from build123d import *

# Parameters (mm, degrees)
EXTRUDE_DEPTH = 50


with BuildPart() as part:
    # Sketch → Extrude (new body)
    with BuildSketch(Plane.XY):
        with BuildLine():
            Line((0, 0), (200, 0))
            Line((200, 0), (200, 11))
            ThreePointArc((200, 11), (197.363961, 17.363961), (191, 20))
            Line((191, 20), (38, 20))
            ThreePointArc((20, 38), (25.272078, 25.272078), (38, 20))
            Line((20, 191), (20, 38))
            ThreePointArc((20, 191), (17.363961, 197.363961), (11, 200))
            Line((0, 200), (11, 200))
            Line((0, 0), (0, 200))
        make_face()
    extrude(amount=EXTRUDE_DEPTH)


solid = part.part
Source: CAD feature listing. Evaluate the final solid. Frame: model axes, mm. A direction names the side the tool comes from. Coordinates: 2 decimals unless noted, no trailing zeros. Loops run counter-clockwise (first coordinate to the right, second up) from the corner with the lowest first, then second, coordinate; pieces in that order, holes last. Notation, with made-up numbers: (56, 55.5) - (91, 55.5) arc R12 cw to (91, 69.5) - close; hole circle Ø10 at (83.5, 42). An arc over 180 degrees is marked (long way). Return JSON: item names as keys, results as strings.
Q1. Section A-A, the plane z = 18.5. Return loops of the section in (x, y), plus the area to 3 significant figures.
Results:
{"outline": "(0, 0) - (200, 0) - (200, 11) arc R9 ccw to (191, 20) - (38, 20) arc R18 cw to (20, 38) - (20, 191) arc R9 ccw to (11, 200) - (0, 200) - close", "area": "7,630 mm2"}
Q2. Access query for faces 1 (the flat face through (0, 99, 25)), 2 (the flat face through (116, 20, 25)). Directions: +Z, -Z, +X, -X, +Y, -Y. A direction counts if a zero-diameter tool reaches every point of the face in a straight line with its end or side. Return the directions, or none.
Results:
{"face 1": "+Z, -Z, -X, +Y, -Y", "face 2": "+Z, -Z, +X, +Y"}
Q3. Material intervals for line 1 along X through (y, z) = (160, 8.5); line 2 along X through (y, z) = (16, 12), sorted ascending.
Results:
{"line 1": "0 to 20", "line 2": "0 to 198.48"}
Q4. Section B-B, the plane x = 87. Return loops of the section in (y, z).
Results:
{"outline": "(0, 0) - (20, 0) - (20, 50) - (0, 50) - close"}
Q5. Contact query for flat-ended pins moving along their axis: P1, Ø10, axis at x = 36, z = 30.5, coming from the +Y side; P2, Ø4, axis at x = 160.5, z = 11.5, coming from the +Y side; P3, Ø3, axis at x = 78, z = 32.5, coming from the -Y side; P4, Ø6, axis at y = 126, z = 34.5, coming from the +X side. Output: stop coordinate, or through.
Results:
{"P1": "y = 21.42", "P2": "y = 20", "P3": "y = 0", "P4": "x = 20"}
